```python
from build123d import *

# Parameters (mm, degrees)
SKETCH1_W           = 241
SKETCH1_H           = 303
BOSS_EXTRUDE1_DEPTH = 10
CUT_EXTRUDE1_DEPTH  = 388.285424461
SKETCH3_R           = 1.5
CUT_EXTRUDE2_DEPTH  = 10


with BuildPart() as part:
    # Sketch1 → Boss-Extrude1 (new body)
    with BuildSketch(Plane(origin=(0, 0, 0), x_dir=(1, 0, 0), z_dir=(0, 1, 0))):
        with Locations((120.5, 151.5)):
            Rectangle(SKETCH1_W, SKETCH1_H)
    extrude(amount=BOSS_EXTRUDE1_DEPTH)

    # Sketch2 → Cut-Extrude1 (cut, through all)
    with BuildSketch(Plane(origin=(0, 10, 0), x_dir=(1, 0, 0), z_dir=(0, 1, 0))):
        with BuildLine():
            Line((50.5, 150), (190.5, 150))
            ThreePointArc((190.5, 150), (194.035533906, 148.535533906), (195.5, 145))
            Line((195.5, 145), (195.5, 135))
            ThreePointArc((195.5, 135), (196.964466094, 131.464466094), (200.5, 130))
            Line((200.5, 130), (210.5, 130))
            ThreePointArc((210.5, 130), (214.035533906, 128.535533906), (215.5, 125))
            Line((215.5, 125), (215.5, 55))
            ThreePointArc((215.5, 55), (214.035533906, 51.464466094), (210.5, 50))
            Line((210.5, 50), (200.5, 50))
            ThreePointArc((200.5, 50), (196.964466094, 48.535533906), (195.5, 45))
            Line((195.5, 45), (195.5, 35))
            ThreePointArc((195.5, 35), (194.035533906, 31.464466094), (190.5, 30))
            Line((190.5, 30), (50.5, 30))
            ThreePointArc((50.5, 30), (46.964466094, 31.464466094), (45.5, 35))
            Line((45.5, 35), (45.5, 45))
            ThreePointArc((45.5, 45), (44.035533906, 48.535533906), (40.5, 50))
            Line((40.5, 50), (30.5, 50))
            ThreePointArc((30.5, 50), (26.964466094, 51.464466094), (25.5, 55))
            Line((25.5, 55), (25.5, 125))
            ThreePointArc((25.5, 125), (26.964466094, 128.535533906), (30.5, 130))
            Line((30.5, 130), (40.5, 130))
            ThreePointArc((40.5, 130), (44.035533906, 131.464466094), (45.5, 135))
            Line((45.5, 135), (45.5, 145))
            ThreePointArc((45.5, 145), (46.964466094, 148.535533906), (50.5, 150))
        make_face()
    extrude(amount=-CUT_EXTRUDE1_DEPTH, mode=Mode.SUBTRACT)

    # Sketch3 → Cut-Extrude2 (cut)
    with BuildSketch(Plane(origin=(0, 10, 0), x_dir=(1, 0, 0), z_dir=(0, 1, 0))):
        with Locations(Location((205.5, 140, 0), (0, 0, 270))):
            Circle(SKETCH3_R)
        with Locations(Location((35.5, 140, 0), (0, 0, 270))):
            Circle(SKETCH3_R)
        with Locations(Location((35.5, 40, 0), (0, 0, 270))):
            Circle(SKETCH3_R)
        with Locations(Location((205.5, 40, 0), (0, 0, 270))):
            Circle(SKETCH3_R)
    extrude(amount=-CUT_EXTRUDE2_DEPTH, mode=Mode.SUBTRACT)


solid = part.part
```
Can you work these out from the model? Positions are in its coordinate system, mm. A direction names the side the tool comes from. Give positions to 0.01 mm unless a question says otherwise; leave off trailing zeros. Write each loop counter-clockwise with the first axis right and the second up, starting at its lowest first coordinate (ties: lowest second). Pieces come first, ordered by that corner, then holes. Notation, with made-up numbers: (55.5, 45.5) -> (66.5, 45.5) arc R26 ccw to (66.5, 66.5) -> close; hole circle Ø10 at (32, 44). An arc over 180 degrees is marked (long way). Write item = value, one per line.
(1) I need wall thicknesses on probe 1 along X at (y, z) = (6, -140); probe 2 along Z at (x, y) = (205.5, 5.5); probe 3 along Z at (x, y) = (123, 1.75). Which ranges of each line are inside material? Lowest first, please. Write a range as from..to.
Worked out:
probe_1 = 0..34, 37..45.5, 195.5..204, 207..241
probe_2 = -303..-141.5, -138.5..-130, -50..-41.5, -38.5..0
probe_3 = -303..-150, -30..0
(2) For faces 4 (the face through (36, 5, -50)), 5 (the face through (119, 10, -187)), which set-ups out of +Z, -Z, +X, -X, +Y, -Y let a thin tool reach every point of the face, with its end or its side?
Worked out:
face_4 = +Y, -Y
face_5 = +Z, -Z, +X, -X, +Y
(3) Thinking about a two-plate mould opening in Z: for faces 1 (the face through (119, 5, -303)), 2 (the face through (119, 0, -187)), 3 (the face through (121, 5, -30)), which applies, released by +Z, released by -Z, zero draft, split by the parting line, or undercut?
Worked out:
face_1 = released by -Z
face_2 = zero draft
face_3 = undercut
(4) Suppose I cut it at A-A on x = 175. Write out the boundary of the cut face in (y, z), then the cut area to 3 significant figures.
Worked out:
outline = (0, -303) -> (10, -303) -> (10, -150) -> (0, -150) -> close; (0, -30) -> (10, -30) -> (10, 0) -> (0, 0) -> close
area = 1,830 mm^2
(5) Suppose I cut it at B-B on y = 6.5. Count the separate pieces of the cut face and the enclosed holes in it, then the cut area to 3 significant figures.
Worked out:
separate_pieces = 1
enclosed_holes = 5
area = 51,800 mm^2
(6) I'm going to push flat-ended pins straight in: P1, Ø2.5, axis at x = 35.5, z = -40, coming from the -Y side; P2, Ø2, axis at y = 1.5, z = -69, coming from the -X side. Where does each tip first touch, or does it pass through?
Worked out:
P1 = through
P2 = 0
